Source: CAD feature listing. Evaluate the final solid. Frame: model axes, mm. Give positions to 0.01 mm unless a question says otherwise; leave off trailing zeros. Loops run counter-clockwise (first coordinate to the right, second up) from the corner with the lowest first, then second, coordinate; pieces in that order, holes last.
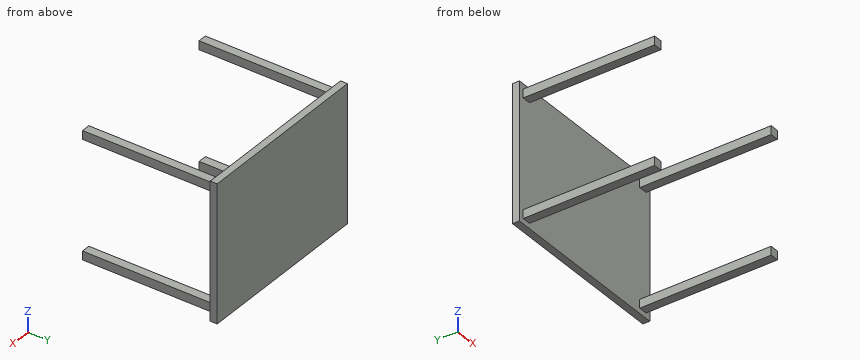
from build123d import *

# Parameters (mm, degrees)
SKETCH1_W           = 1040
SKETCH1_H           = 790
BOSS_EXTRUDE1_DEPTH = 20
SKETCH2_W           = 50
SKETCH2_H           = 50
BOSS_EXTRUDE2_DEPTH = 760


with BuildPart() as part:
    # Sketch1 → Boss-Extrude1 (new, symmetric)
    with BuildSketch(Plane(origin=(0, 0, 0), x_dir=(1, 0, 0), z_dir=(0, 1, 0))):
        Rectangle(SKETCH1_W, SKETCH1_H)
    extrude(amount=BOSS_EXTRUDE1_DEPTH, both=True)

    # Sketch2 → Boss-Extrude2 (add)
    with BuildSketch(Plane.XZ.offset(20)):
        with Locations((-465, 340)):
            Rectangle(SKETCH2_W, SKETCH2_H)
        with Locations((-465, -340)):
            Rectangle(SKETCH2_W, SKETCH2_H)
        with Locations((465, -340)):
            Rectangle(SKETCH2_W, SKETCH2_H)
        with Locations((465, 340)):
            Rectangle(SKETCH2_W, SKETCH2_H)
    extrude(amount=BOSS_EXTRUDE2_DEPTH)


solid = part.part
1) Cut plane B-B (z = 116.5). Return loops of the section in (x, y).
Checks:
outline: (-520, -20) - (520, -20) - (520, 20) - (-520, 20) - close
2) Cut plane C-C (x = -47). Return loops of the section in (y, z).
Checks:
outline: (-20, -395) - (20, -395) - (20, 395) - (-20, 395) - close
3) Cut plane A-A (y = -544). Return loops of the section in (x, z), and give its area (3 significant figures).
Checks:
outline: (-490, -365) - (-440, -365) - (-440, -315) - (-490, -315) - close; (-490, 315) - (-440, 315) - (-440, 365) - (-490, 365) - close; (440, -365) - (490, -365) - (490, -315) - (440, -315) - close; (440, 315) - (490, 315) - (490, 365) - (440, 365) - close
area: 10,000 mm2
4) Contact query for flat-ended pins moving along their axis: P1, Ø15, axis at y = -238, z = -334, coming from the -X side; P2, Ø15, axis at x = 467.5, y = -544.5, coming from the +Z side; P3, Ø25, axis at y = -495, z = -333, coming from the +X side. Output: stop coordinate, or through.
Checks:
P1: stops at x = -490
P2: stops at z = 365
P3: stops at x = 490
5) Ray query, probe 1 along Z at (x, y) = (-463, -225.5); probe 2 along X at (y, z) = (-438, 344); probe 3 along Y at (x, z) = (36, 277.5). Return the intervals inside material, ascending.
Checks:
probe 1: z = -365 to -315, 315 to 365
probe 2: x = -490 to -440, 440 to 490
probe 3: y = -20 to 20
